Model file for the job. Use its own axes, mm. A direction names the side the tool comes from. Coordinates: 2 decimals unless noted, no trailing zeros. Loops run counter-clockwise (first coordinate to the right, second up) from the corner with the lowest first, then second, coordinate; pieces in that order, holes last. Notation, with made-up numbers: M 32,-19.75 L 48,-19.75 A36 cw 48,17.25 Z; hole C 23,63.5 d10. An arc over 180 degrees is marked long. One line per question, with ' | ' between items. Start each with the question number.
Solid Edge part; units mm, degrees
sketch "Sketch1" plane through (0, 0, 0) normal (0, 0, 1) x (1, 0, 0)
  circle A0 centre (0, 0) radius 9.525
extrude "Protrusion1" add sketch "Sketch1" along normal blind 7.9248
sketch "Sketch2" plane through (0, 0, 0) normal (0, 0, -1) x (0, 1, 0)
  circle A0 centre (0, 0) radius 6.35
extrude "Protrusion2" add sketch "Sketch2" along normal blind 101.6
sketch "Sketch3" plane through (0, 0, -101.6) normal (0, 0, -1) x (0, 1, 0)
  circle A0 centre (0, 0) radius 4.7625
extrude "Protrusion3" add sketch "Sketch3" along normal blind 15.875
sketch "Sketch4" plane through (0, 0, 7.9248) normal (0, 0, 1) x (0, 1, 0)
  line L0 (-3.175, 1.7461) -> (0, 3.8287)
  line L1 (-3.175, -2.051) -> (-3.175, 1.7461)
  line L2 (-3.175, -2.051) -> (0, -3.8287)
  line L3 (3.175, -2.051) -> (0, -3.8287)
  line L4 (3.175, -2.051) -> (3.175, 1.7461)
  line L5 (3.175, 1.7461) -> (0, 3.8287)
extrude "Cutout1" cut sketch "Sketch4" against normal blind 3.9624
chamfer "Chamfer1" distance 0.7874 angle 45 1 edges at (0, -4.7625, -117.475)
properties part number "144841"
(1) Two-plate mould, pull along Y, no slides. Class faces 4 (the face through (4, 0, 7.925)), 5 (the face through (0, -3.175, 6)), 6 (the face through (2.9, -3.78, -109.04)): pulls with the +Y half, pulls with the -Y half, needs draft (parallel to the pull), parting line crosses it, or undercut.
(2) Pin check, flat tips, straight feed: P1, Ø1, axis at y = -4, z = -75, coming from the -X side; P2, Ø1.5, axis at y = 0, z = -24.5, coming from the +X side; P3, Ø5, axis at y = -3.5, z = -87.5, coming from the -X side; P4, Ø1.1, axis at x = 0.5, z = 5, coming from the +Y side (3 decimals). Stop position of each tip, or through.
(3) Band-saw the part on B-B on z = -10. Write the cut outline in (x, y).
(4) 3-axis set-ups, long thin cutter, end or side, ignore diameter. For faces 1 (the face through (-2.773, -1.61, 5.971)), 2 (the face through (6.2, -2, 0)), 3 (the face through (-7.559, 5.796, 3.907)): which of +Z, -Z, +X, -X, +Y, -Y reach the whole face in a straight line?
(5) Drill centre lines: line 1 (Z direction, x = -0.5, y = -2.75) (3 decimals); line 2 (Z direction, x = -0.25, y = 8.5); line 3 (Y direction, x = -4.75, z = -38.5). Where is each one in solid material? Low to high. Write a range as [from, to].
Computed values:
1) face 4: needs draft | face 5: undercut | face 6: parting line crosses it
2) P1: x = -5.3 | P2: x = 6.35 | P3: x = -6.27 | P4: y = 9.525
3) outline: C 0,0 d12.7
4) face 1: +Z | face 2: -Z | face 3: +Z, -Z
5) line 1: [-117.475, 3.962] | line 2: [0, 7.92] | line 3: [-4.21, 4.21]
